Read the model definition and answer for the solid it produces. Units are mm, in the model's axes. Face numbers are marked on the shaded views. A direction names the side the tool comes from. Give positions to 0.01 mm unless a question says otherwise; leave off trailing zeros. Loops run counter-clockwise (first coordinate to the right, second up) from the corner with the lowest first, then second, coordinate; pieces in that order, holes last. Notation, with made-up numbers: (-34.75, -24) - (21.25, -24) arc R19 cw to (21.25, -17) - close; hole circle Ø3 at (69, 7). An arc over 180 degrees is marked (long way). Put each result on its own line as item: value. Start each with the question number.
1. For the marked faces 1, 2, 3 and 4, determine the directions among +Z, -Z, +X, -X, +Y, -Y from which every point of the face is accessible in a straight line to the end or side of a thin tool.
2. Consider L1, parallel to X at y = -0.5, z = 12.5; L2, parallel to Z at x = -6.75, y = 1.25; L3, parallel to Z at x = 2.5, y = -3.25. Determine where each line is inside the solid, lowest interval first. Write a range as from..to.
3. A cutting plane is placed at B-B, the plane y = 0. Determine the outline of the cut face in (x, z) (3 decimals), plus the area to 3 significant figures.
4. Given pin 1 Ø2 at (y, z) = (0, 8.5) entering from +X; pin 2 Ø8 at (y, z) = (-2.5, 20.5) entering from -X; pin 3 Ø5 at (x, y) = (3, 2.5) entering from -Z; pin 4 Ø1.5 at (x, z) = (-5, 4.5) entering from +Y, each flat-ended and moving along its own axis, determine where each tip first touches the part or whether it passes through.
5. A cutting plane is placed at A-A, the plane x = 0. Determine the outline of the cut face in (y, z) (3 decimals), plus the area to 3 significant figures.
6. A cutting plane is placed at C-C, the plane z = 8.5. Determine the outline of the cut face in (x, y), plus the area to 3 significant figures.
7. A cutting plane is placed at D-D, the plane y = -3.75. Determine the outline of the cut face in (x, z), plus the area to 3 significant figures.
```python
from build123d import *

# Parameters (mm, degrees)
F0_R     = 8.32
F1_DEPTH = 3.2
F3_DEPTH = 20.8
F4_R     = 3.175
F5_DEPTH = 9


with BuildPart() as f1:
    # F0 (on Top) → F1 (new body)
    with BuildSketch(Plane.XY):
        Circle(F0_R)
    extrude(amount=F1_DEPTH)

    # F2 (on face) → F3 (join)
    with BuildSketch(Plane.XY.offset(3.2)):
        with BuildLine():
            Line((5.1, -2.204975), (5.1, 2.204975))
            ThreePointArc((5.1, 2.204975), (0, 5.55625), (-5.1, 2.204975))
            Line((-5.1, 2.204975), (-5.1, -2.204975))
            ThreePointArc((-5.1, -2.204975), (0, -5.55625), (5.1, -2.204975))
        make_face()
    extrude(amount=F3_DEPTH)

    # F4 (on face) → F5 (join)
    with BuildSketch(Plane(origin=(0, 0, 0), x_dir=(1, 0, 0), z_dir=(0, 0, -1))):
        Circle(F4_R)
    extrude(amount=F5_DEPTH)


solid = f1.part
```
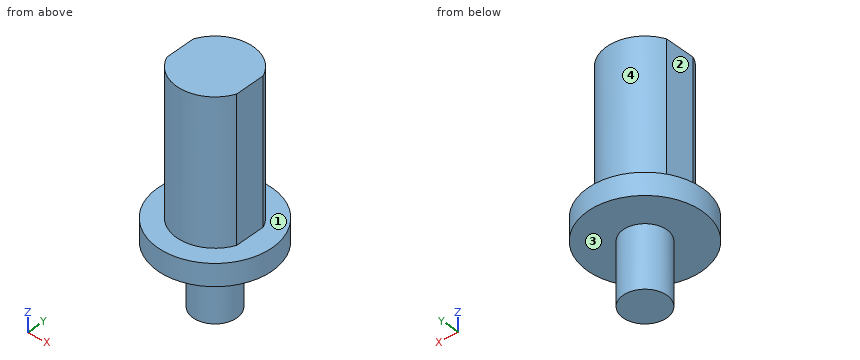
Return value:
1. face 1: +Z
1. face 2: +Z, -X, +Y, -Y
1. face 3: -Z
1. face 4: +Z, +Y
2. L1: x = -5.1..5.1
2. L2: z = 0..3.2
2. L3: z = 0..24
3. outline: (-8.32, 0) - (-3.175, 0) - (-3.175, -9) - (3.175, -9) - (3.175, 0) - (8.32, 0) - (8.32, 3.2) - (5.1, 3.2) - (5.1, 24) - (-5.1, 24) - (-5.1, 3.2) - (-8.32, 3.2) - close
3. area: 323 mm2
4. pin 1: stops at x = 5.1
4. pin 2: stops at x = -5.1
4. pin 3: stops at z = -9
4. pin 4: stops at y = 3.58
5. outline: (-8.32, 0) - (-3.175, 0) - (-3.175, -9) - (3.175, -9) - (3.175, 0) - (8.32, 0) - (8.32, 3.2) - (5.556, 3.2) - (5.556, 24) - (-5.556, 24) - (-5.556, 3.2) - (-8.32, 3.2) - close
5. area: 342 mm2
6. outline: (-5.1, -2.2) arc R5.56 ccw to (5.1, -2.2) - (5.1, 2.2) arc R5.56 ccw to (-5.1, 2.2) - close
6. area: 94.3 mm2
7. outline: (-7.43, 0) - (7.43, 0) - (7.43, 3.2) - (4.1, 3.2) - (4.1, 24) - (-4.1, 24) - (-4.1, 3.2) - (-7.43, 3.2) - close
7. area: 218 mm2
